from build123d import *

# Parameters (mm, degrees)
SKETCH1_W                  = 35
SKETCH1_H                  = 10
BOSS_EXTRUDE1_DEPTH        = 7
SKETCH2_W                  = 20
SKETCH2_H                  = 10
BOSS_EXTRUDE2_DEPTH        = 5
FILLET1_R                  = 0.5
F_3_6_3_6_DIAMETER_HOLE1_D = 3.6


with BuildPart() as part:
    # Sketch1 → Boss-Extrude1 (new body)
    with BuildSketch(Plane.XY):
        Rectangle(SKETCH1_W, SKETCH1_H)
    extrude(amount=BOSS_EXTRUDE1_DEPTH)

    # Sketch2 → Boss-Extrude2 (add)
    with BuildSketch(Plane(origin=(0, 0, 0), x_dir=(-1, 0, 0), z_dir=(0, 0, -1))):
        with Locations((7.5, 0)):
            Rectangle(SKETCH2_W, SKETCH2_H)
    extrude(amount=BOSS_EXTRUDE2_DEPTH)

    # Fillet1
    fillet1_edges = [part.edges().sort_by_distance(p)[0] for p in [
        (10, -5, 0),
        (2.5, 5, -2.5),
        (2.5, -5, -2.5),
        (0, -5, 7),
        (-7.5, 5, -5),
        (-7.5, -5, -5),
        (10, 5, 0),
        (0, 5, 7),
    ]]
    fillet(fillet1_edges, radius=FILLET1_R)

    # Ø3.6 (3.6) Diameter Hole1 (through all)
    with Locations(Plane(origin=(-12, 0, 7), x_dir=(1, 0, 0), z_dir=(0, 0, 1))):
        with Locations((0, 0)):
            Hole(F_3_6_3_6_DIAMETER_HOLE1_D / 2)


solid = part.part
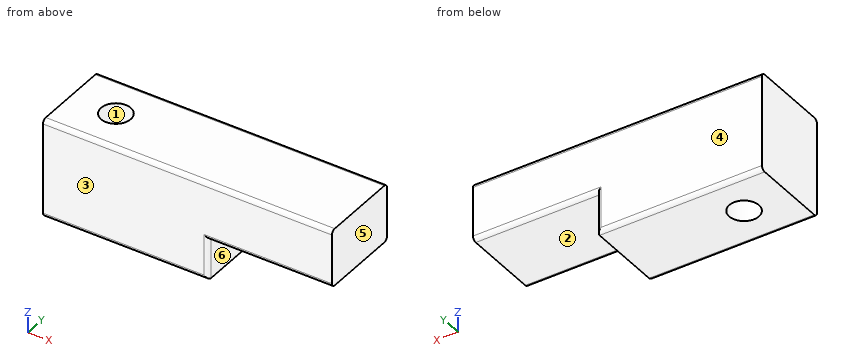
For this review, take the finished solid that the model builds, in its own axes (mm). Face numbers are marked on the shaded views. A direction names the side the tool comes from. Coordinates: 2 decimals unless noted, no trailing zeros. Loops run counter-clockwise (first coordinate to the right, second up) from the corner with the lowest first, then second, coordinate; pieces in that order, holes last. Notation, with made-up numbers: (64.25, -17.75) - (94.25, -17.75) arc R9 cw to (94.25, -5.75) - close; hole circle Ø2 at (26.5, 61). An arc over 180 degrees is marked (long way). Use a Markdown table: item, result. Add a question column.
Item 1: We need section B-B (x = -12). Give the boundary of the cut face in (y, z), and give its area (3 significant figures).
Item 2: We need section D-D (y = -3). Give the boundary of the cut face in (x, z), and give its area (3 significant figures).
Item 3: Mouldability with a two-part tool opening along Y and no side actions: class the marked faces 1, 2, 3 and 4 as pulls with the +Y half, pulls with the -Y half, needs draft (parallel to the pull), parting line crosses it, or undercut.
Item 4: Insertion check: pin 1 Ø2.5 at (x, y) = (13.5, -0.5) entering from -Z; pin 2 Ø1.5 at (y, z) = (1.5, -3.5) entering from +X. Each pin has a flat end and moves straight along its axis. Give the tip position at first contact, or say it passes through.
Item 5: We need section C-C (y = 0). Give the boundary of the cut face in (x, z), and give its area (3 significant figures).
Item 6: For line 1 (Y direction, x = -12, z = 3); line 2 (X direction, y = 2.75, z = -1.25); line 3 (Z direction, x = 12.5, y = 3.5), list the stretches that pass through material, from the lowest coordinate up.
Item 7: Tool access review of the marked faces 5 and 6: name each direction out of +Z, -Z, +X, -X, +Y, -Y from which nothing blocks a thin tool from reaching the whole face with its end or side.
Item 8: We need section A-A (z = 5.25). Give the boundary of the cut face in (x, y), and give its area (3 significant figures).
Results list:
| question | item | result |
|---|---|---|
| 1 | outline | (-5, -4.5) arc R0.5 ccw to (-4.5, -5) - (-1.8, -5) - (-1.8, 7) - (-4.5, 7) arc R0.5 ccw to (-5, 6.5) - close; (1.8, -5) - (4.5, -5) arc R0.5 ccw to (5, -4.5) - (5, 6.5) arc R0.5 ccw to (4.5, 7) - (1.8, 7) - close |
| 1 | area | 76.6 mm^2 |
| 2 | outline | (-17.5, -5) - (2.5, -5) - (2.5, 0) - (17.5, 0) - (17.5, 7) - (-17.5, 7) - close |
| 2 | area | 345 mm^2 |
| 3 | face 1 | undercut |
| 3 | face 2 | needs draft |
| 3 | face 3 | pulls with the -Y half |
| 3 | face 4 | pulls with the +Y half |
| 4 | pin 1 | stops at z = 0 |
| 4 | pin 2 | stops at x = 2.5 |
| 5 | outline | (-17.5, -5) - (-13.8, -5) - (-13.8, 7) - (-17.5, 7) - close; (-10.2, -5) - (2.5, -5) - (2.5, 0) - (17.5, 0) - (17.5, 7) - (-10.2, 7) - close |
| 5 | area | 302 mm^2 |
| 6 | line 1 | y = -5 to -1.8, 1.8 to 5 |
| 6 | line 2 | x = -17.5 to 2.5 |
| 6 | line 3 | z = 0 to 7 |
| 7 | face 5 | +Z, -Z, +X, +Y, -Y |
| 7 | face 6 | -Z, +X, +Y, -Y |
| 8 | outline | (-17.5, -5) - (17.5, -5) - (17.5, 5) - (-17.5, 5) - close; hole circle Ø3.6 at (-12, 0) |
| 8 | area | 340 mm^2 |
